from build123d import *

# Parameters (mm, degrees)
SKETCH1_W               = 20.5
SKETCH1_H               = 45.4
EXTRUDE1_DEPTH          = 1.75
SKETCH2_R               = 0.75
CUT_EXTRUDE1_DEPTH      = 1.75
MIRROR2_COPY_1_SKETCH_R = 0.75
MIRROR2_COPY_1_DEPTH    = 1.75


with BuildPart() as part:
    # Sketch1 → Extrude1 (new body)
    with BuildSketch(Plane.XY):
        Rectangle(SKETCH1_W, SKETCH1_H)
    extrude(amount=EXTRUDE1_DEPTH)

    # Sketch2 → Cut-Extrude1 (cut)
    with BuildSketch(Plane.XY.offset(1.75)):
        with Locations((8.75, -21.2)):
            Circle(SKETCH2_R)
    cut_extrude1 = extrude(amount=-CUT_EXTRUDE1_DEPTH, mode=Mode.SUBTRACT)

    # Mirror1: Cut-Extrude1 across plane
    add(cut_extrude1.mirror(Plane(origin=(0, 0, 0), x_dir=(0, 0, 1), z_dir=(1, 0, 0))), mode=Mode.SUBTRACT)

    # Mirror2: Cut-Extrude1 across plane
    add(cut_extrude1.mirror(Plane.ZX), mode=Mode.SUBTRACT)

    # Mirror2 copy 1 sketch → Mirror2 copy 1 (cut)
    with BuildSketch(Plane(origin=(0, 0, 1.75), x_dir=(-1, 0, 0), z_dir=(0, 0, 1))):
        with Locations((8.75, -21.2)):
            Circle(MIRROR2_COPY_1_SKETCH_R)
    extrude(amount=-MIRROR2_COPY_1_DEPTH, mode=Mode.SUBTRACT)


solid = part.part
Source: CAD feature listing. Evaluate the final solid. Frame: model axes, mm. Give positions to 0.01 mm unless a question says otherwise; leave off trailing zeros. Write each loop counter-clockwise with the first axis right and the second up, starting at its lowest first coordinate (ties: lowest second). Pieces come first, ordered by that corner, then holes. Notation, with made-up numbers: (-34.75, 70.5) -> (-24.75, 70.5) arc R31 cw to (-24.75, 109.5) -> close; hole circle Ø9 at (80.25, 20). An arc over 180 degrees is marked (long way). Write item = value, one per line.
Q1. Cut plane A-A on y = 21.2. Return loops of the section in (x, z), then the cut area to 3 significant figures.
Here are the results:
outline = (-10.25, 0) -> (-9.5, 0) -> (-9.5, 1.75) -> (-10.25, 1.75) -> close; (-8, 0) -> (8, 0) -> (8, 1.75) -> (-8, 1.75) -> close; (9.5, 0) -> (10.25, 0) -> (10.25, 1.75) -> (9.5, 1.75) -> close
area = 30.6 mm²
Q2. Line query: line 1 (Y direction, x = 8.75, z = 1.1); line 2 (X direction, y = 21.2, z = 0.45); line 3 (Y direction, x = 8.25, z = 1.5). Output: solid intervals per line, ascending. Write a range as from..to.
Here are the results:
line_1 = -22.7..-21.95, -20.45..20.45, 21.95..22.7
line_2 = -10.25..-9.5, -8..8, 9.5..10.25
line_3 = -22.7..-21.76, -20.64..20.64, 21.76..22.7
Q3. Cut plane B-B on x = 8.75. Return loops of the section in (y, z), then the cut area to 3 significant figures.
Here are the results:
outline = (-22.7, 0) -> (-21.95, 0) -> (-21.95, 1.75) -> (-22.7, 1.75) -> close; (-20.45, 0) -> (20.45, 0) -> (20.45, 1.75) -> (-20.45, 1.75) -> close; (21.95, 0) -> (22.7, 0) -> (22.7, 1.75) -> (21.95, 1.75) -> close
area = 74.2 mm²
Q4. First-contact query: pin 1 (2 mm diameter, centred on x = 8.75, y = 21.2, fed in from +Z). Flat tip, straight axial feed; report the tip coordinate or a pass-through.
Here are the results:
pin_1 = 1.75
Q5. Mould query, pull axis Y, two halves, no side actions, for faces 1 (the face through (0, 22.7, 1)), 2 (the face through (8.2, -20.69, 0.89)), 3 (the face through (0, -22.7, 1)), 4 (the face through (0, 0, 0)). Classes: +Y half, -Y half, draft (parallel to the pull), parting line (faces both ways), or undercut.
Here are the results:
face_1 = +Y half
face_2 = undercut
face_3 = -Y half
face_4 = draft
